from build123d import *

# Parameters (mm, degrees)
F0_W     = 123.4
F0_H     = 244.057946
F1_DEPTH = 3.55
F2_T     = -2.54
F4_R     = 5
F3_R     = 2.602058
F5_DEPTH = 25


with BuildPart() as f1:
    # F0 (on Front) → F1 (new body, symmetric)
    with BuildSketch(Plane.XZ):
        Rectangle(F0_W, F0_H)
    extrude(amount=F1_DEPTH, both=True)

    # F2
    f2_openings = [f1.faces().sort_by_distance(p)[0] for p in [
        (0, -3.55, 0),
    ]]
    offset(amount=F2_T, openings=f2_openings)

    # F4
    f4_edges = [f1.edges().sort_by_distance(p)[0] for p in [
        (61.7, 0, 122.028973),
        (-61.7, 0, 122.028973),
        (-61.7, 0, -122.028973),
        (61.7, 0, -122.028973),
    ]]
    fillet(f4_edges, radius=F4_R)

    # F3 (on Front) → F5 (cut)
    with BuildSketch(Plane.XZ):
        with BuildLine():
            ThreePointArc((25.559906, 51.782791), (20.077513, 56.652751), (15.887922, 50.634407))
            ThreePointArc((15.887922, 50.634407), (21.233963, 46.91283), (25.559906, 51.782791))
        make_face()
        with Locations((6.310866, 50.634407)):
            Circle(F3_R)
    extrude(amount=-F5_DEPTH, mode=Mode.SUBTRACT)


solid = f1.part
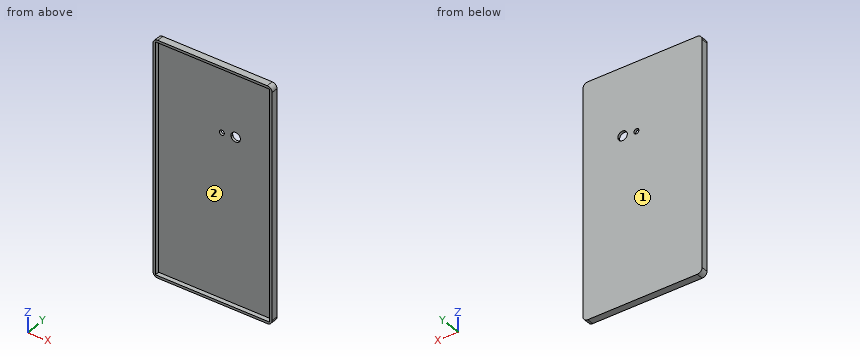
Geometry: final body of the model. Coordinates: model frame, mm. Face numbers are marked on the shaded views. Round coordinates to 2 decimals unless told otherwise and drop trailing zeros. Order: outer loops, then holes, each group sorted by start corner. A loop starts at its lowest first (then second) coordinate and runs counter-clockwise, first axis right, second up. Notation, with made-up numbers: (55.25, 88.5) -> (99.25, 88.5) arc R29 ccw to (99.25, 116.5) -> close; hole circle Ø3 at (-3, -13). An arc over 180 degrees is marked (long way). Put each result on its own line as item: value. Start each with the question number.
Q1. Line query: probe 1 along Z at (x, y) = (-8, -1.5); probe 2 along X at (y, z) = (-1, -25); probe 3 along Y at (x, z) = (-50.5, 19). Output: solid intervals per line, ascending.
Q2. First-contact query: pin 1 (3 mm diameter, centred on x = 6.31, z = 50.63, fed in from -Y); pin 2 (3 mm diameter, centred on x = 40, z = -15.5, fed in from -Y). Flat tips, straight axial feed; report the tip coordinate or a pass-through.
Q3. Section C-C on z = 78.5. Return the cut outline in (x, y).
Q4. Section A-A on y = -1.25. Return the cut outline in (x, z), and give its area (3 significant figures).
Q5. Pull-direction query (X, two-part tool) for the marked faces 1 and 2; classes: +X half, -X half, draft (parallel to the pull), parting line (faces both ways), or undercut.
Q6. Section B-B on x = -14. Return the cut outline in (y, z).
Ans:
1. probe 1: z = -122.03 to -119.49, 119.49 to 122.03
1. probe 2: x = -61.7 to -59.16, 59.16 to 61.7
1. probe 3: y = 1.01 to 3.55
2. pin 1: passes through
2. pin 2: stops at y = 1.01
3. outline: (-61.7, -3.55) -> (-59.16, -3.55) -> (-59.16, 1.01) -> (59.16, 1.01) -> (59.16, -3.55) -> (61.7, -3.55) -> (61.7, 3.55) -> (-61.7, 3.55) -> close
4. outline: (-61.7, -117.03) arc R5 ccw to (-56.7, -122.03) -> (56.7, -122.03) arc R5 ccw to (61.7, -117.03) -> (61.7, 117.03) arc R5 ccw to (56.7, 122.03) -> (-56.7, 122.03) arc R5 ccw to (-61.7, 117.03) -> close; hole (-59.16, -119.49) -> (59.16, -119.49) -> (59.16, 119.49) -> (-59.16, 119.49) -> close
4. area: 1,820 mm2
5. face 1: draft
5. face 2: undercut
6. outline: (-3.55, -122.03) -> (3.55, -122.03) -> (3.55, 122.03) -> (-3.55, 122.03) -> (-3.55, 119.49) -> (1.01, 119.49) -> (1.01, -119.49) -> (-3.55, -119.49) -> close
